Here's how the part is built. I have some questions about the finished solid (model axes, mm). Round coordinates to 2 decimals unless told otherwise and drop trailing zeros. Loops run counter-clockwise (first coordinate to the right, second up) from the corner with the lowest first, then second, coordinate; pieces in that order, holes last. Notation, with made-up numbers: M 1,79 L 40,79 A5 cw 40,86 Z; hole C -3.5,23 d6. An arc over 180 degrees is marked long. Answer as a JSON object with one key per item and string values.
from build123d import *

# Parameters (mm, degrees)
F2_DEPTH  = 17.5
F3_DEPTH  = 17.5
F4_W      = 35
F4_H      = 17.5
F5_DEPTH  = 35
F6_W      = 35
F6_H      = 17.5
F7_DEPTH  = 35
F8_W      = 35
F8_H      = 17.5
F9_DEPTH  = 35
F10_W     = 35
F10_H     = 17.5
F11_DEPTH = 35


with BuildPart() as f2:
    # F0 (on Front) → F2 (new body, symmetric)
    with BuildSketch(Plane.XZ):
        Polygon((700, 150), (-700, 150), (-600, -150), (600, -150), align=None)
    extrude(amount=F2_DEPTH, both=True)

    # F1 (on face) → F3 (cut, symmetric)
    with BuildSketch(Plane.XZ):
        Polygon((651.440094, 115), (-651.440094, 115), (-574.773427, -115), (574.773427, -115), align=None)
    extrude(amount=F3_DEPTH, both=True, mode=Mode.SUBTRACT)

    # F4 (on face) → F5 (cut)
    with BuildSketch(Plane.XZ.offset(17.5)):
        with Locations((-417.5, -123.75)):
            Rectangle(F4_W, F4_H)
    extrude(amount=-F5_DEPTH, mode=Mode.SUBTRACT)

    # F6 (on face) → F7 (cut)
    with BuildSketch(Plane.XZ.offset(17.5)):
        with Locations((417.5, -123.75)):
            Rectangle(F6_W, F6_H)
    extrude(amount=-F7_DEPTH, mode=Mode.SUBTRACT)

    # F8 (on face) → F9 (cut)
    with BuildSketch(Plane.XZ.offset(17.5)):
        with Locations((-417.5, 123.75)):
            Rectangle(F8_W, F8_H)
    extrude(amount=-F9_DEPTH, mode=Mode.SUBTRACT)

    # F10 (on face) → F11 (cut)
    with BuildSketch(Plane.XZ.offset(17.5)):
        with Locations((417.5, 123.75)):
            Rectangle(F10_W, F10_H)
    extrude(amount=-F11_DEPTH, mode=Mode.SUBTRACT)


solid = f2.part
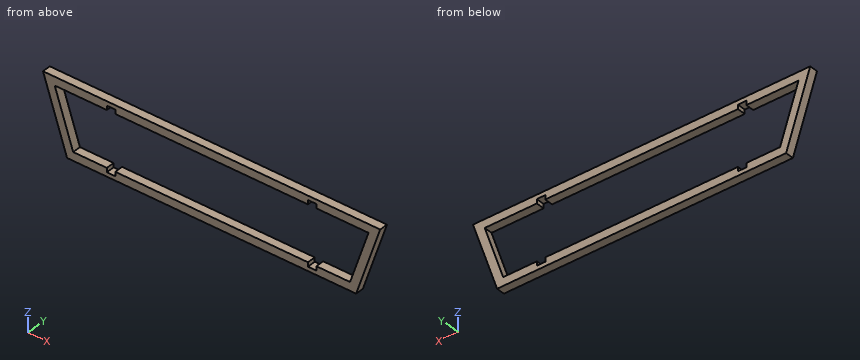
Item 1: I want a section at A-A on x = 147. List the corners of the cut face in (y, z) for me, plus the area to 3 significant figures.
Solution:
{"outline": "M -17.5,-150 L 17.5,-150 L 17.5,-115 L -17.5,-115 Z; M -17.5,115 L 17.5,115 L 17.5,150 L -17.5,150 Z", "area": "2,450 mm2"}
Item 2: I want a section at B-B on y = 0. List the corners of the cut face in (x, z) for me, plus the area to 3 significant figures.
Solution:
{"outline": "M -700,150 L -600,-150 L 600,-150 L 700,150 Z; hole M -651.44,115 L -574.77,-115 L -435,-115 L -435,-132.5 L -400,-132.5 L -400,-115 L 400,-115 L 400,-132.5 L 435,-132.5 L 435,-115 L 574.77,-115 L 651.44,115 L 435,115 L 435,132.5 L 400,132.5 L 400,115 L -400,115 L -400,132.5 L -435,132.5 L -435,115 Z", "area": "106,000 mm2"}
Item 3: If I drill on L1, parallel to Z at x = -373.5, y = -9.5; L2, parallel to Z at x = -424.5, y = -3.5; L3, parallel to X at y = 7.5, z = 120, over which ranges is the centre line in solid material (lowest first)? Write a range as from..to.
Solution:
{"L1": "z = -150..-115, 115..150", "L2": "z = -150..-132.5, 132.5..150", "L3": "x = -690..-435, -400..400, 435..690"}
Item 4: I want a section at C-C on x = 417. List the corners of the cut face in (y, z) for me.
Solution:
{"outline": "M -17.5,-150 L 17.5,-150 L 17.5,-132.5 L -17.5,-132.5 Z; M -17.5,132.5 L 17.5,132.5 L 17.5,150 L -17.5,150 Z"}
Item 5: For P1, Ø10, axis at y = -2.5, z = -3, coming from the +X side; P2, Ø19, axis at y = -1.5, z = -126.5, coming from the +X side; P3, Ø19, axis at y = 1.5, z = 126, coming from the +X side, each with a flat end and sliding along its axis, tell me the tip position at first contact or that it passes through.
Solution:
{"P1": "stops at x = 650.67", "P2": "stops at x = 611", "P3": "stops at x = 695.17"}
